```python
from build123d import *

# Parameters (mm, degrees)
SKETCH1_R              = 6.2
SKETCH1_R_2            = 1.25
MAIN_DEPTH             = 1.5
SKETCH2_W              = 35
SKETCH2_H              = 16
FRAMEWORK_DEPTH        = 3
SKETCH3_R              = 1.5
FIXHOLE_DEPTH          = 7
HOLEPATTERN_COUNT      = 2
HOLEPATTERN_PITCH      = 25
HOLEPATTERN_COUNT_DIR2 = 2
HOLEPATTERN_PITCH_DIR2 = 10
CUT_EXTRUDE1_REACH     = 23
SKETCH4_R              = 15


with BuildPart() as part:
    # Sketch1 → Main (new body, symmetric)
    with BuildSketch(Plane.XY):
        with BuildLine():
            Line((-39.3, 10.723805295), (-39.3, -10.723805295))
            ThreePointArc((-39.3, -10.723805295), (-35.08887909, -13.155479355), (-30.3, -14))
            Line((-30.3, -14), (30.3, -14))
            ThreePointArc((30.3, -14), (35.08887909, -13.155479355), (39.3, -10.723805295))
            Line((39.3, -10.723805295), (39.3, 10.723805295))
            ThreePointArc((39.3, 10.723805295), (35.08887909, 13.155479355), (30.3, 14))
            Line((30.3, 14), (-30.3, 14))
            ThreePointArc((-30.3, 14), (-35.08887909, 13.155479355), (-39.3, 10.723805295))
        make_face()
        with Locations((-30.3, 0)):
            Circle(SKETCH1_R, mode=Mode.SUBTRACT)
        with Locations((-35.3, 10)):
            Circle(SKETCH1_R_2, mode=Mode.SUBTRACT)
        with Locations((-25.3, 10)):
            Circle(SKETCH1_R_2, mode=Mode.SUBTRACT)
        with Locations((-35.3, -10)):
            Circle(SKETCH1_R_2, mode=Mode.SUBTRACT)
        with Locations((-25.3, -10)):
            Circle(SKETCH1_R_2, mode=Mode.SUBTRACT)
        with Locations((30.3, 0)):
            Circle(SKETCH1_R, mode=Mode.SUBTRACT)
        with Locations((25.3, 10)):
            Circle(SKETCH1_R_2, mode=Mode.SUBTRACT)
        with Locations((35.3, 10)):
            Circle(SKETCH1_R_2, mode=Mode.SUBTRACT)
        with Locations((25.3, -10)):
            Circle(SKETCH1_R_2, mode=Mode.SUBTRACT)
        with Locations((35.3, -10)):
            Circle(SKETCH1_R_2, mode=Mode.SUBTRACT)
    extrude(amount=MAIN_DEPTH, both=True)

    # Sketch2 → Framework (add)
    with BuildSketch(Plane(origin=(0, 0, 1.5), x_dir=(-1, 0, 0), z_dir=(0, 0, -1))):
        Polygon((21.3, 14), (10, 14), (10, 7), (-10, 7), (-10, 14), (-21.3, 14), (-21.3, -14), (21.3, -14), align=None)
        with Locations((0, -3)):
            Rectangle(SKETCH2_W, SKETCH2_H, mode=Mode.SUBTRACT)
    extrude(amount=-FRAMEWORK_DEPTH)

    # Sketch3 → FixHole (cut, through all)
    with BuildSketch(Plane(origin=(0, 0, -1.5), x_dir=(-1, 0, 0), z_dir=(0, 0, -1))):
        with Locations((12.5, -8)):
            Circle(SKETCH3_R)
    fixhole = extrude(amount=-FIXHOLE_DEPTH, mode=Mode.SUBTRACT)

    # HolePattern: FixHole 2 × 2
    with Locations(*[(i * HOLEPATTERN_PITCH, j * HOLEPATTERN_PITCH_DIR2, 0) for i in range(HOLEPATTERN_COUNT) for j in range(HOLEPATTERN_COUNT_DIR2) if (i, j) != (0, 0)]):
        add(fixhole, mode=Mode.SUBTRACT)

    # Sketch4 → Cut-Extrude1 (cut, up to next)
    with BuildSketch(Plane(origin=(0, 7, 0), x_dir=(1, 0, 0), z_dir=(0, 1, 0)), mode=Mode.PRIVATE) as cut_extrude1_sk1:
        with Locations((0, -16.5)):
            Circle(SKETCH4_R)
    cut_extrude1_tool1 = extrude(cut_extrude1_sk1.sketch, amount=-CUT_EXTRUDE1_REACH, mode=Mode.PRIVATE) & part.part
    add(cut_extrude1_tool1.solids().sort_by_distance((0, 7, 16.5))[0], mode=Mode.SUBTRACT)


solid = part.part
```
Model file for the job. Use its own axes, mm. A direction names the side the tool comes from. Round coordinates to 2 decimals unless told otherwise and drop trailing zeros. Write each loop counter-clockwise with the first axis right and the second up, starting at its lowest first coordinate (ties: lowest second). Pieces come first, ordered by that corner, then holes. Notation, with made-up numbers: (42, 67.25) - (46, 67.25) arc R21 ccw to (46, 91.25) - close; hole circle Ø7 at (30.5, 72.25). An arc over 180 degrees is marked (long way). One line per item, written item: value.
(1) Cut at C-C, the plane x = -12.5. Give the cut face in (y, z).
Values follow:
outline: (-14, -1.5) - (-9.5, -1.5) - (-9.5, 1.5) - (-11, 1.5) - (-11, 4.5) - (-14, 4.5) - close; (-6.5, -1.5) - (0.5, -1.5) - (0.5, 1.5) - (-6.5, 1.5) - close; (3.5, -1.5) - (14, -1.5) - (14, 4.5) - (5, 4.5) - (5, 1.5) - (3.5, 1.5) - close
(2) Drop flat-ended pins along their axis: P1, Ø3.5, axis at y = 5, z = 3, coming from the +X side; P2, Ø5.5, axis at x = 34.5, y = -0.5, coming from the +Z side; P3, Ø0.9, axis at y = -6, z = 2.5, coming from the -X side. Give the stop position or say it passes through.
Values follow:
P1: stops at x = 39.3
P2: stops at z = 1.5
P3: stops at x = -21.3
(3) Cut at D-D, the plane x = -31.5. Give the cut face in (y, z), plus the area to 3 significant figures.
Values follow:
outline: (-13.95, -1.5) - (-6.08, -1.5) - (-6.08, 1.5) - (-13.95, 1.5) - close; (6.08, -1.5) - (13.95, -1.5) - (13.95, 1.5) - (6.08, 1.5) - close
area: 47.2 mm²
(4) Wall check: probe 1 along Y at (x, z) = (12.5, -0.25); probe 2 along X at (y, z) = (-10, 3.75); probe 3 along Y at (x, z) = (12.5, 2). Give the ranges that are in metal, low to high.
Values follow:
probe 1: y = -14 to -9.5, -6.5 to 0.5, 3.5 to 14
probe 2: x = -21.3 to -17.5, 17.5 to 21.3
probe 3: y = -14 to -11, 5 to 14
(5) 3-axis set-ups, long thin cutter, end or side, ignore diameter. For faces 5 (the flat face through (0, -3, 1.5)), 6 (the flat face through (28, -6, 1.5)), 7 (the flat face through (-10, 11, 3)): which of +Z, -Z, +X, -X, +Y, -Y reach the whole face in a straight line?
Values follow:
face 5: +Z
face 6: +Z, +X, +Y, -Y
face 7: +Z, +Y
(6) Cut at A-A, the plane z = 0. Give the number of separate pieces and of enclosed holes in the cut face, plus the area to 3 significant figures.
Values follow:
separate pieces: 1
enclosed holes: 14
area: 1,850 mm²
(7) Cut at B-B, the plane y = -8. Give the cut face in (x, z), plus the area to 3 significant figures.
Values follow:
outline: (-39.3, -1.5) - (-14, -1.5) - (-14, 1.5) - (-17.5, 1.5) - (-17.5, 4.5) - (-21.3, 4.5) - (-21.3, 1.5) - (-39.3, 1.5) - close; (-11, -1.5) - (11, -1.5) - (11, 1.5) - (-11, 1.5) - close; (14, -1.5) - (39.3, -1.5) - (39.3, 1.5) - (21.3, 1.5) - (21.3, 4.5) - (17.5, 4.5) - (17.5, 1.5) - (14, 1.5) - close
area: 241 mm²
(8) Two-plate mould, pull along X, no slides. Class faces 1 (the flat face through (0, -14, 2)), 2 (the flat face through (-17.5, -3, 3)), 3 (the cylindrical face through (-24.11, 10.38, -0.02)), 4 (the flat face through (-21.3, 0, 3)): pulls with the +X half, pulls with the -X half, needs draft (parallel to the pull), parting line crosses it, or undercut.
Values follow:
face 1: needs draft
face 2: undercut
face 3: undercut
face 4: pulls with the -X half
